from build123d import *

# Parameters (mm, degrees)
F1_DEPTH = 71.12
F2_W     = 1.27
F2_H     = 1.27
F3_DEPTH = 6.35
F4_W     = 2.54
F4_H     = 2.54
F5_DEPTH = 17.77746


with BuildPart() as f1:
    # F0 (on Front) → F1 (new body)
    with BuildSketch(Plane.XZ):
        Polygon((8.5148252547, 76.2), (0, 0), (15.24, 0), align=None)
    extrude(amount=F1_DEPTH)

    # F2 (on face) → F3 (join)
    with BuildSketch(Plane(origin=(0, 0, 0), x_dir=(1, 0, 0), z_dir=(0, 0, -1))):
        with Locations((8.255, 42.545)):
            Rectangle(F2_W, F2_H)
        with Locations((8.255, 43.815)):
            Rectangle(F2_W, F2_H)
        with Locations((6.985, 43.815)):
            Rectangle(F2_W, F2_H)
        with Locations((6.985, 42.545)):
            Rectangle(F2_W, F2_H)
        with Locations((8.255, 28.575)):
            Rectangle(F2_W, F2_H)
        with Locations((6.985, 28.575)):
            Rectangle(F2_W, F2_H)
        with Locations((6.985, 27.305)):
            Rectangle(F2_W, F2_H)
        with Locations((8.255, 27.305)):
            Rectangle(F2_W, F2_H)
    extrude(amount=F3_DEPTH)

    # F4 (on face) → F5 (join)
    with BuildSketch(Plane.XZ.offset(44.45)):
        with Locations((7.62, -5.08)):
            Rectangle(F4_W, F4_H)
    extrude(amount=-F5_DEPTH)


solid = f1.part
Could you check a few things on this model? Use its own coordinates, in mm. A direction names the side the tool comes from. Give positions to 0.01 mm unless a question says otherwise; leave off trailing zeros. Order: outer loops, then holes, each group sorted by start corner. A loop starts at its lowest first (then second) coordinate and runs counter-clockwise, first axis right, second up.
1. For faces 4 (the flat face through (6.35, -36, -5)), 5 (the flat face through (8.89, -35, -5)), 6 (the flat face through (8, -36, -3.81)), which set-ups out of +Z, -Z, +X, -X, +Y, -Y let a thin tool reach every point of the face, with its end or its side?
2. Suppose I cut it at C-C (y = -12.5). List the corners of the cut face in (x, z) for me, plus the area to 3 significant figures.
3. We'd pull the mould along Z, two halves only. Please class faces 1 (the flat face through (8, -29.21, -2)), 2 (the flat face through (8, -44.45, -3)), 3 (the flat face through (11.924, -35.062, 37.567)): pulls with the +Z half, pulls with the -Z half, needs draft (parallel to the pull), parting line crosses it, or undercut.
4. Will these pins go through, and if not, where does the flat tip stop? P1, Ø3, axis at y = -50, z = 5, coming from the +X side; P2, Ø2, axis at x = 7.5, z = -1.5, coming from the -Y side; P3, Ø4, axis at x = 3.5, y = -28, coming from the -Z side.
5. I need wall thicknesses on L1, parallel to X at y = -67, z = 16; L2, parallel to X at y = -3.5, z = 27.5. Which ranges of each line are inside material? Lowest first, please.
6. Suppose I cut it at D-D (x = 11). List the corners of the cut face in (y, z) for me.
7. Suppose I cut it at A-A (y = -33.5). List the corners of the cut face in (x, z) for me.
8. Suppose I cut it at B-B (z = 5). List the corners of the cut face in (x, y) for me.
Solved:
1. face 4: -Z, -X, +Y, -Y
1. face 5: -Z, +X, +Y, -Y
1. face 6: +X, -X
2. outline: (0, 0) - (15.24, 0) - (8.51, 76.2) - close
2. area: 581 mm2
3. face 1: undercut
3. face 2: needs draft
3. face 3: pulls with the +Z half
4. P1: stops at x = 14.93
4. P2: stops at y = -44.45
4. P3: stops at z = 0
5. L1: x = 1.79 to 13.83
5. L2: x = 3.07 to 12.81
6. outline: (-71.12, 0) - (0, 0) - (0, 48.04) - (-71.12, 48.04) - close
7. outline: (0, 0) - (15.24, 0) - (8.51, 76.2) - close; (6.35, -6.35) - (8.89, -6.35) - (8.89, -3.81) - (6.35, -3.81) - close
8. outline: (0.56, -71.12) - (14.8, -71.12) - (14.8, 0) - (0.56, 0) - close
